The model under review builds one solid part; all positions refer to its coordinate system, in mm. A direction names the side the tool comes from. Give positions to 0.01 mm unless a question says otherwise; leave off trailing zeros. Order: outer loops, then holes, each group sorted by start corner. A loop starts at its lowest first (then second) coordinate and runs counter-clockwise, first axis right, second up.
```python
from build123d import *

# Parameters (mm, degrees)
SKETCH1_R                 = 9.5
BOSS_EXTRUDE1_DEPTH       = 5
F_6_0MM_DOWEL_HOLE1_D     = 6
M3X0_5_TAPPED_HOLE1_D     = 2.5
M3X0_5_TAPPED_HOLE2_D     = 2.5
M3X0_5_TAPPED_HOLE2_DEPTH = 10
M3X0_5_TAPPED_HOLE2_TIP   = 0.751075774


with BuildPart() as part:
    # Sketch1 → Boss-Extrude1 (new body)
    with BuildSketch(Plane(origin=(0, 0, 0), x_dir=(1, 0, 0), z_dir=(0, 1, 0))):
        with Locations(Location((0, 0, 0), (0, 0, 270))):
            Circle(SKETCH1_R)
    extrude(amount=BOSS_EXTRUDE1_DEPTH)

    # Ø6.0mm Dowel Hole1 (through all)
    with Locations(Plane(origin=(0, 5, 0), x_dir=(1, 0, 0), z_dir=(0, 1, 0))):
        with Locations((0, 0)):
            Hole(F_6_0MM_DOWEL_HOLE1_D / 2)

    # M3x0.5 Tapped Hole1 (through all)
    with Locations(Plane(origin=(0, 5, 0), x_dir=(1, 0, 0), z_dir=(0, 1, 0))):
        with Locations((4.490128061, 4.490128061), (-4.490128061, 4.490128061), (-4.490128061, -4.490128061), (4.490128061, -4.490128061)):
            Hole(M3X0_5_TAPPED_HOLE1_D / 2)

    # M3x0.5 Tapped Hole2
    with Locations(Plane(origin=(0, 2.5, 9.5), x_dir=(1, 0, 0), z_dir=(0, 0, 1))):
        with Locations((0, 0)):
            Hole(M3X0_5_TAPPED_HOLE2_D / 2, depth=M3X0_5_TAPPED_HOLE2_DEPTH)
            with Locations((0, 0, -(M3X0_5_TAPPED_HOLE2_DEPTH + M3X0_5_TAPPED_HOLE2_TIP / 2))):  # 118° drill point
                Cone(0, M3X0_5_TAPPED_HOLE2_D / 2, M3X0_5_TAPPED_HOLE2_TIP, mode=Mode.SUBTRACT)


solid = part.part
```
Item 1: Clearance check with flat-ended pins moving along their axes: pin 1 Ø1.5 at (x, z) = (4.49, 4.49) entering from +Y; pin 2 Ø2 at (y, z) = (4, 2.5) entering from -X; pin 3 Ø1.5 at (x, y) = (0, 2.5) entering from +Z. State where each tip first meets the part, or that it passes through.
Values found:
pin 1: passes through
pin 2: stops at x = -9.38
pin 3: stops at z = -2.9
Item 2: For faces 1 (the cylindrical face through (0.16, 3.74, 6.07)), 2 (the cylindrical face through (0, 2, -3)), list the 3-axis set-ups (+Z, -Z, +X, -X, +Y, -Y) from which the entire face can be reached by the end or side of a thin tool; tool diameter is ignored.
Values found:
face 1: +Z
face 2: +Y, -Y
Item 3: Take a section at D-D (x = 0). Give the boundary of the cut face in (y, z).
Values found:
outline: (0, -9.5) - (5, -9.5) - (5, -3) - (0, -3) - close; (0, 3) - (1.25, 3) - (1.25, 9.5) - (0, 9.5) - close; (3.75, 3) - (5, 3) - (5, 9.5) - (3.75, 9.5) - close
Item 4: Take a section at A-A (z = 0). Give the boundary of the cut face in (x, y), and give its area (3 significant figures).
Values found:
outline: (-9.5, 0) - (-3, 0) - (-3, 5) - (-9.5, 5) - close; (3, 0) - (9.5, 0) - (9.5, 5) - (3, 5) - close
area: 65.0 mm2
Item 5: Take a section at C-C (y = 0.3). Give the boundary of the cut face in (x, z).
Values found:
outline: circle Ø19 at (0, 0); hole circle Ø2.5 at (-4.49, -4.49); hole circle Ø2.5 at (-4.49, 4.49); hole circle Ø6 at (0, 0); hole circle Ø2.5 at (4.49, -4.49); hole circle Ø2.5 at (4.49, 4.49)
Item 6: Draft analysis for pull direction X (two halves, no side actions). For faces 3 (the cylindrical face through (-5.78, 2.46, -7.54)), 4 (the cylindrical face through (5.74, 2.46, -4.55)), 5 (the flat face through (2.24, 0, -2.24)), state which applies: released by +X, released by -X, zero draft, split by the parting line, or undercut.
Values found:
face 3: split by the parting line
face 4: undercut
face 5: zero draft
Item 7: Take a section at B-B (x = -4.25). Give the boundary of the cut face in (y, z).
Values found:
outline: (0, -8.5) - (5, -8.5) - (5, -5.72) - (0, -5.72) - close; (0, -3.26) - (5, -3.26) - (5, 3.26) - (0, 3.26) - close; (0, 5.72) - (5, 5.72) - (5, 8.5) - (0, 8.5) - close
Item 8: For line 1 (Y direction, x = 0, z = 4); line 2 (Z direction, x = 5.5, y = 2.4); line 3 (Z direction, x = 4.5, y = 4.5), list the stretches that pass through material, from the lowest coordinate up.
Values found:
line 1: y = 0 to 1.25, 3.75 to 5
line 2: z = -7.75 to -5.23, -3.75 to 3.75, 5.23 to 7.75
line 3: z = -8.37 to -5.74, -3.24 to 3.24, 5.74 to 8.37
